Work out the finished part from the listing and answer in its coordinate system (mm). A direction names the side the tool comes from. Coordinates: 2 decimals unless noted, no trailing zeros. Loops run counter-clockwise (first coordinate to the right, second up) from the corner with the lowest first, then second, coordinate; pieces in that order, holes last. Notation, with made-up numbers: (24, 65.5) -> (35, 65.5) arc R31 ccw to (35, 94.5) -> close; hole circle Ø1 at (86, 70.25). An arc over 180 degrees is marked (long way). Use a Markdown table: item, result.
from build123d import *

# Parameters (mm, degrees)
SKETCH1_R           = 3
BOSS_EXTRUDE1_DEPTH = 8
SKETCH2_R           = 2.5
CUT_EXTRUDE1_DEPTH  = 3
CUT_EXTRUDE2_START  = -2
SKETCH3_R           = 2.5
CUT_EXTRUDE2_DEPTH  = 2
SKETCH4_R           = 2.5
BOSS_EXTRUDE2_DEPTH = 10
SKETCH5_R           = 3
SKETCH5_R_2         = 2.5
BOSS_EXTRUDE3_DEPTH = 10


with BuildPart() as part:
    # Sketch1 → Boss-Extrude1 (new body)
    with BuildSketch(Plane(origin=(0, 0, 0), x_dir=(0, 0, -1), z_dir=(1, 0, 0))):
        Circle(SKETCH1_R)
    extrude(amount=BOSS_EXTRUDE1_DEPTH)

    # Sketch2 → Cut-Extrude1 (cut)
    with BuildSketch(Plane(origin=(8, 0, 0), x_dir=(0, 0, -1), z_dir=(1, 0, 0))):
        Circle(SKETCH2_R)
    extrude(amount=-CUT_EXTRUDE1_DEPTH, mode=Mode.SUBTRACT)

    # Sketch3 → Cut-Extrude2 (cut)
    with BuildSketch(Plane.ZY.offset(CUT_EXTRUDE2_START)):
        with Locations(Location((0, 0, 0), (0, 0, 180))):
            Circle(SKETCH3_R)
    extrude(amount=CUT_EXTRUDE2_DEPTH, mode=Mode.SUBTRACT)

    # Sketch4 → Boss-Extrude2 (add)
    with BuildSketch(Plane.ZY.offset(-2)):
        with Locations(Location((0, 0, 0), (0, 0, 180))):
            Circle(SKETCH4_R)
    extrude(amount=BOSS_EXTRUDE2_DEPTH)

    # Sketch5 → Boss-Extrude3 (add)
    with BuildSketch(Plane.ZY):
        Circle(SKETCH5_R)
        with Locations(Location((0, 0, 0), (0, 0, 180))):
            Circle(SKETCH5_R_2, mode=Mode.SUBTRACT)
    extrude(amount=BOSS_EXTRUDE3_DEPTH)


solid = part.part
Q1. Section C-C on x = -5 is taken. Determine the outline of the cut face in (y, z), and give its area (3 significant figures).
Solved:
| item | result |
|---|---|
| outline | circle Ø6 at (0, 0) |
| area | 28.3 mm² |
Q2. Given pin 1 Ø2 at (x, z) = (-8, -0.5) entering from +Y; pin 2 Ø1.5 at (y, z) = (1, 0.5) entering from -X, each flat-ended and moving along its own axis, determine where each tip first touches the part or whether it passes through.
Solved:
| item | result |
|---|---|
| pin 1 | y = 3 |
| pin 2 | x = -8 |
Q3. Section A-A on y = 0 is taken. Determine the outline of the cut face in (x, z), and give its area (3 significant figures).
Solved:
| item | result |
|---|---|
| outline | (-10, -3) -> (8, -3) -> (8, -2.5) -> (5, -2.5) -> (5, 2.5) -> (8, 2.5) -> (8, 3) -> (-10, 3) -> (-10, 2.5) -> (-8, 2.5) -> (-8, -2.5) -> (-10, -2.5) -> close |
| area | 83.0 mm² |
Q4. Consider line 1 (Y direction, x = -9.4, z = 0); line 2 (X direction, y = 2.1, z = -0.3); line 3 (Y direction, x = 1.25, z = 0.1). Determine where each line is inside the solid, lowest interval first. Write a range as [from, to].
Solved:
| item | result |
|---|---|
| line 1 | [-3, -2.5], [2.5, 3] |
| line 2 | [-8, 5] |
| line 3 | [-3, 3] |
Q5. For faces 1 (the cylindrical face through (-9, -0.1, 2.5)), 2 (the cylindrical face through (6.52, -2.44, 0.54)), 3 (the flat face through (-10, 2, -2)), determine the directions among +Z, -Z, +X, -X, +Y, -Y from which every point of the face is accessible in a straight line to the end or side of a thin tool.
Solved:
| item | result |
|---|---|
| face 1 | -X |
| face 2 | +X |
| face 3 | +Z, -Z, -X, +Y, -Y |
Q6. Determine the mould class of faces 4 (the flat face through (8, 2, 2)), 5 (the flat face through (-8, 0, 0)) for opening direction Y: pulls with the +Y half, pulls with the -Y half, needs draft (parallel to the pull), parting line crosses it, or undercut.
Solved:
| item | result |
|---|---|
| face 4 | needs draft |
| face 5 | undercut |
